from build123d import *

# Parameters (mm, degrees)
SKETCH_3_W               = 120
SKETCH_3_H               = 60
EXTRUDE_2_DEPTH          = 16
FILLET_3_R               = 19
SKETCH_4_R               = 29
EXTRUDE_3_DEPTH          = 60
CUT_EXTRUDE_1_DEPTH      = 168.931533668
CUT_EXTRUDE_1_DEPTH_BACK = 168.931533668
SKETCH_5_R               = 18
EXTRUDE_4_REACH          = 172.985
EXTRUDE_4_END_RADIUS     = 29
SKETCH_9_R               = 14
CUT_EXTRUDE_2_REACH      = 172.985
CUT_EXTRUDE_2_END_RADIUS = 18
SKETCH_10_R              = 8
EXTRUDE_8_DEPTH          = 12
RIB_26_REACH             = 137.779
SKETCH_14_WALL_W         = 300.558465316
SKETCH_14_WALL_H         = 12
CUT_EXTRUDE_3_DEPTH      = 173.06103578


with BuildPart() as part:
    # Sketch 3 → Extrude 2 (new body)
    with BuildSketch(Plane(origin=(0, 0, 0), x_dir=(1, 0, 0), z_dir=(0, 1, 0))):
        with Locations((60, -30)):
            Rectangle(SKETCH_3_W, SKETCH_3_H)
    extrude(amount=EXTRUDE_2_DEPTH)

    # Fillet 3
    fillet_3_edges = [part.edges().sort_by_distance(p)[0] for p in [
        (120, 8, 60),
        (0, 8, 60),
    ]]
    fillet(fillet_3_edges, radius=FILLET_3_R)



with BuildPart() as body_2:
    # Sketch 4 → Extrude 3 (new body)
    with BuildSketch(Plane(origin=(0, 0, -3), x_dir=(-1, 0, 0), z_dir=(0, 0, -1))):
        with Locations((-60, 72)):
            Circle(SKETCH_4_R)
    extrude(amount=-EXTRUDE_3_DEPTH)

    # Sketch 5 → Cut-Extrude 1 (cut, two sides: drawn at the far end of the back side and taken through both)
    with BuildSketch(Plane.XY.offset(57).offset(-CUT_EXTRUDE_1_DEPTH_BACK)):
        with Locations((60, 72)):
            Circle(SKETCH_5_R)
    extrude(amount=CUT_EXTRUDE_1_DEPTH + CUT_EXTRUDE_1_DEPTH_BACK, mode=Mode.SUBTRACT)

    # Extrude 4: up to this cylinder (the profile starts outside it)
    extrude_4_end = Plane(origin=(60, 72, 27), z_dir=(0, 0, -1)) * Cylinder(EXTRUDE_4_END_RADIUS, 404.97, mode=Mode.PRIVATE)
    # Sketch 9 → Extrude 4 (add, up to the surface)
    with BuildSketch(Plane(origin=(0, 106, 0), x_dir=(1, 0, 0), z_dir=(0, 1, 0)), mode=Mode.PRIVATE) as extrude_4_sk1:
        with Locations(Location((60, -27, 0), (0, 0, 270))):
            Circle(SKETCH_9_R)
    extrude_4_tool1 = extrude(extrude_4_sk1.sketch, amount=-EXTRUDE_4_REACH, mode=Mode.PRIVATE) - extrude_4_end
    add(extrude_4_tool1.solids().sort_by_distance((60, 106, 27))[0])

    # Cut-Extrude 2: up to this cylinder (the profile starts outside it)
    cut_extrude_2_end = Plane(origin=(60, 72, 27), z_dir=(0, 0, 1)) * Cylinder(CUT_EXTRUDE_2_END_RADIUS, 382.97, mode=Mode.PRIVATE)
    # Sketch 10 → Cut-Extrude 2 (cut, up to the surface)
    with BuildSketch(Plane(origin=(0, 106, 0), x_dir=(1, 0, 0), z_dir=(0, 1, 0)), mode=Mode.PRIVATE) as cut_extrude_2_sk1:
        with Locations(Location((60, -27, 0), (0, 0, 270))):
            Circle(SKETCH_10_R)
    cut_extrude_2_tool1 = extrude(cut_extrude_2_sk1.sketch, amount=-CUT_EXTRUDE_2_REACH, mode=Mode.PRIVATE) - cut_extrude_2_end
    add(cut_extrude_2_tool1.solids().sort_by_distance((60, 106, 27))[0], mode=Mode.SUBTRACT)


with BuildPart() as part_1:
    add(part.part)

    add(body_2.part)  # Extrude 8 merges body 2
    # Sketch 11 → Extrude 8 (add)
    with BuildSketch(Plane.XY):
        with BuildLine():
            ThreePointArc((33.99807912, 84.841343799), (60, 43), (86.00192088, 84.841343799))
            Line((86.00192088, 84.841343799), (120, 16))
            Line((120, 16), (0, 16))
            Line((0, 16), (33.99807912, 84.841343799))
        make_face()
    extrude(amount=EXTRUDE_8_DEPTH)

    # Sketch 14 wall → Rib 26 (add, up to next)
    with BuildSketch(Plane(origin=(60, 29.5, 48), x_dir=(0, 1, 0), z_dir=(0, 0, 1)), mode=Mode.PRIVATE) as rib_26_sk1:
        Rectangle(SKETCH_14_WALL_W, SKETCH_14_WALL_H)
    rib_26_tool1 = extrude(rib_26_sk1.sketch, amount=-RIB_26_REACH, mode=Mode.PRIVATE) - part_1.part
    add(rib_26_tool1.solids().sort_by_distance((60, 29.5, 48))[0])

    # Sketch 16 → Cut-Extrude 3 (cut, through all)
    with BuildSketch(Plane.XY.offset(60)):
        Polygon((33, 0), (33, 2), (87, 2), (87, 0), (60, 0), align=None)
    extrude(amount=-CUT_EXTRUDE_3_DEPTH, mode=Mode.SUBTRACT)

    # Sketch 20 → M18 _C_1 (revolve, cut)
    with BuildSketch(Plane(origin=(101, 16, 41), x_dir=(0, 0, 1), z_dir=(1, 0, 0))):
        Polygon((0, 0), (0, 16), (10, 16), (10, 0.5), (18, 0.5), (18, 0.020977491), (18.025, 0), align=None)
    revolve(axis=Axis((101, 22.35, 41), (0, -1, 0)), mode=Mode.SUBTRACT)

    # Sketch 22 → M18 _C_2 (revolve, cut)
    with BuildSketch(Plane(origin=(19, 0, 41), x_dir=(0, 0, -1), z_dir=(1, 0, 0))):
        Polygon((0, 0), (0, 106), (10, 106), (10, 0.5), (18, 0.5), (18, 0.020977491), (18.025, 0), align=None)
    revolve(axis=Axis((19, -6.35, 41), (0, 1, 0)), mode=Mode.SUBTRACT)


solid = part_1.part
The listing builds one solid part. Answer for the finished solid, in the listing's coordinates (mm). A direction names the side the tool comes from. Round coordinates to 2 decimals unless told otherwise and drop trailing zeros. Order: outer loops, then holes, each group sorted by start corner. A loop starts at its lowest first (then second) coordinate and runs counter-clockwise, first axis right, second up. Notation, with made-up numbers: (-13.5, 84) - (31.5, 84) arc R26 ccw to (31.5, 98) - close; hole circle Ø1 at (66, 67). An arc over 180 degrees is marked (long way). Write item = value, one per line. Start each with the question number.
1) Section A-A, the plane x = 60 is taken. Write down the section's boundary in (y, z), plus the area to 3 significant figures.
2) Section C-C, the plane z = 2 is taken. Write down the section's boundary in (x, y), plus the area to 3 significant figures.
3) For faces 1 (the cylindrical face through (46.62, 46.27, 26.58)), 2 (the cylindrical face through (54.638, 102.715, 39.932)), 3 (the flat face through (66, 30, 30)), determine the directions among +Z, -Z, +X, -X, +Y, -Y from which every point of the face is accessible in a straight line to the end or side of a thin tool.
4) Section B-B, the plane y = 65.5 is taken. Write down the section's boundary in (x, z).
5) Straight lines are drawn through the part: L1, parallel to X at y = 10.75, z = 41; L2, parallel to X at y = 0.45, z = 41; L3, parallel to Z at x = 60, y = 92. For each, find the intervals that lie inside material, in ascending order.
6) For a pull along X with two mould halves and no side action, classify faces 4 (the cylindrical face through (114.29, 8.11, 54.58)), 5 (the cylindrical face through (91.085, 7.858, 39.698)), 6 (the flat face through (61, 24, 0)) as released by +X, released by -X, zero draft, split by the parting line, or undercut.
7) Given pin 1 (6 mm diameter, centred on x = 27, z = 33, fed in from -Y); pin 2 (10 mm diameter, centred on x = 70, y = 83, fed in from +Z); pin 3 (21 mm diameter, centred on x = 60, z = 27, fed in from -Y); pin 4 (12 mm diameter, centred on x = 101, z = 41, fed in from -Y), each flat-ended and moving along its own axis, determine where each tip first touches the part or whether it passes through.
8) Section D-D, the plane y = 7 is taken. Write down the section's boundary in (x, z), plus the area to 3 significant figures.
Results list:
q1.outline = (2, 0) - (43, 0) - (43, -3) - (54, -3) - (54, 57) - (43, 57) - (43, 48) - (16, 48) - (16, 60) - (2, 60) - close; (90, -3) - (101, -3) - (101, 13) - (106, 13) - (106, 19) - (90, 19) - close; (90, 35) - (106, 35) - (106, 41) - (101, 41) - (101, 57) - (90, 57) - close
q1.area = 3,340 mm^2
q2.outline = (0, 0) - (33, 0) - (33, 2) - (87, 2) - (87, 0) - (120, 0) - (120, 16) - (86, 84.84) arc R29 ccw to (34, 84.84) - (0, 16) - close; hole circle Ø36 at (60, 72)
q2.area = 7,320 mm^2
q3.face_1 = none
q3.face_2 = +Y
q3.face_3 = +Z, +X
q4.outline = (24.45, 0) - (31.74, 0) - (31.74, -3) - (43.21, -3) - (43.21, 57) - (31.74, 57) - (31.74, 12) - (24.45, 12) - close; (76.79, -3) - (88.26, -3) - (88.26, 0) - (95.55, 0) - (95.55, 12) - (88.26, 12) - (88.26, 57) - (76.79, 57) - close
q5.L1 = 0 to 9, 29 to 91, 111 to 120
q5.L2 = 0 to 1, 87 to 91, 111 to 120
q5.L3 = -3 to 19, 35 to 57
q6.face_4 = released by +X
q6.face_5 = undercut
q6.face_6 = zero draft
q7.pin_1 = 0.5
q7.pin_2 = 57
q7.pin_3 = 2
q7.pin_4 = through
q8.outline = (0, 0) - (120, 0) - (120, 41) arc R19 ccw to (101, 60) - (19, 60) arc R19 ccw to (0, 41) - close; hole circle Ø20 at (19, 41); hole circle Ø20 at (101, 41)
q8.area = 6,420 mm^2
